Read the model definition and answer for the solid it produces. Units are mm, in the model's axes. A direction names the side the tool comes from. Coordinates: 2 decimals unless noted, no trailing zeros. Order: outer loops, then holes, each group sorted by start corner. A loop starts at its lowest first (then second) coordinate and runs counter-clockwise, first axis right, second up. Notation, with made-up numbers: (48, -11) -> (105, -11) arc R16 ccw to (105, 6) -> close; hole circle Ø8 at (-32.5, 54). An arc over 180 degrees is marked (long way). Use CSV: the item, a comma, the result in double quotes.
```python
from build123d import *

# Parameters (mm, degrees)
SKETCH_1_W      = 23
SKETCH_1_H      = 14
SKETCH_1_W_2    = 2
SKETCH_1_W_3    = 0.7
SKETCH_1_H_2    = 0.7
EXTRUDE_1_DEPTH = 1
SKETCH_1_3_W    = 2
SKETCH_1_3_H    = 14
SKETCH_1_3_W_2  = 0.7
SKETCH_1_3_H_2  = 0.7
EXTRUDE_2_DEPTH = 2
SKETCH_1_4_W    = 0.7
SKETCH_1_4_H    = 0.7
EXTRUDE_3_DEPTH = 2.5
SKETCH_1_5_W    = 0.7
SKETCH_1_5_H    = 0.7
EXTRUDE_4_DEPTH = 4
SKETCH_2_W      = 0.7
SKETCH_2_H      = 0.7
EXTRUDE_5_DEPTH = 7
SKETCH_4_W      = 19
SKETCH_4_H      = 12
EXTRUDE_6_DEPTH = 2.5
SKETCH_4_2_W    = 19
SKETCH_4_2_H    = 12
EXTRUDE_7_DEPTH = 1.5


with BuildPart() as part:
    # Sketch 1 → Extrude 1 (new body)
    # profile 1 of 7: a face of its own
    with BuildSketch(Plane.XY):
        with Locations((-13.5, 7)):
            Rectangle(SKETCH_1_W, SKETCH_1_H)
    # profile 2 of 7: a face of its own
    with BuildSketch(Plane.XY):
        with Locations((-1, 7)):
            Rectangle(SKETCH_1_W_2, SKETCH_1_H)
        with Locations((-1, 2)):
            Rectangle(SKETCH_1_W_3, SKETCH_1_H_2, mode=Mode.SUBTRACT)
        with Locations((-1, 4.5)):
            Rectangle(SKETCH_1_W_3, SKETCH_1_H_2, mode=Mode.SUBTRACT)
        with Locations((-1, 7)):
            Rectangle(SKETCH_1_W_3, SKETCH_1_H_2, mode=Mode.SUBTRACT)
        with Locations((-1, 9.5)):
            Rectangle(SKETCH_1_W_3, SKETCH_1_H_2, mode=Mode.SUBTRACT)
        with Locations((-1, 12)):
            Rectangle(SKETCH_1_W_3, SKETCH_1_H_2, mode=Mode.SUBTRACT)
    # profile 3 of 7: a face of its own
    with BuildSketch(Plane.XY):
        with Locations((-1, 12)):
            Rectangle(SKETCH_1_W_3, SKETCH_1_H_2)
    # profile 4 of 7: a face of its own
    with BuildSketch(Plane.XY):
        with Locations((-1, 9.5)):
            Rectangle(SKETCH_1_W_3, SKETCH_1_H_2)
    # profile 5 of 7: a face of its own
    with BuildSketch(Plane.XY):
        with Locations((-1, 7)):
            Rectangle(SKETCH_1_W_3, SKETCH_1_H_2)
    # profile 6 of 7: a face of its own
    with BuildSketch(Plane.XY):
        with Locations((-1, 4.5)):
            Rectangle(SKETCH_1_W_3, SKETCH_1_H_2)
    # profile 7 of 7: a face of its own
    with BuildSketch(Plane.XY):
        with Locations((-1, 2)):
            Rectangle(SKETCH_1_W_3, SKETCH_1_H_2)
    extrude(amount=EXTRUDE_1_DEPTH)

    # Sketch 1_3 → Extrude 2 (add)
    with BuildSketch(Plane.XY):
        with Locations((-1, 7)):
            Rectangle(SKETCH_1_3_W, SKETCH_1_3_H)
        with Locations((-1, 2)):
            Rectangle(SKETCH_1_3_W_2, SKETCH_1_3_H_2, mode=Mode.SUBTRACT)
        with Locations((-1, 4.5)):
            Rectangle(SKETCH_1_3_W_2, SKETCH_1_3_H_2, mode=Mode.SUBTRACT)
        with Locations((-1, 7)):
            Rectangle(SKETCH_1_3_W_2, SKETCH_1_3_H_2, mode=Mode.SUBTRACT)
        with Locations((-1, 9.5)):
            Rectangle(SKETCH_1_3_W_2, SKETCH_1_3_H_2, mode=Mode.SUBTRACT)
        with Locations((-1, 12)):
            Rectangle(SKETCH_1_3_W_2, SKETCH_1_3_H_2, mode=Mode.SUBTRACT)
    extrude(amount=-EXTRUDE_2_DEPTH)

    # Sketch 1_4 → Extrude 3 (add)
    with BuildSketch(Plane.XY):
        with Locations((-1, 12)):
            Rectangle(SKETCH_1_4_W, SKETCH_1_4_H)
        with Locations((-1, 9.5)):
            Rectangle(SKETCH_1_4_W, SKETCH_1_4_H)
        with Locations((-1, 7)):
            Rectangle(SKETCH_1_4_W, SKETCH_1_4_H)
        with Locations((-1, 4.5)):
            Rectangle(SKETCH_1_4_W, SKETCH_1_4_H)
        with Locations((-1, 2)):
            Rectangle(SKETCH_1_4_W, SKETCH_1_4_H)
    extrude(amount=EXTRUDE_3_DEPTH)

    # Sketch 1_5 → Extrude 4 (add)
    with BuildSketch(Plane.XY):
        with Locations((-1, 12)):
            Rectangle(SKETCH_1_5_W, SKETCH_1_5_H)
        with Locations((-1, 9.5)):
            Rectangle(SKETCH_1_5_W, SKETCH_1_5_H)
        with Locations((-1, 7)):
            Rectangle(SKETCH_1_5_W, SKETCH_1_5_H)
        with Locations((-1, 4.5)):
            Rectangle(SKETCH_1_5_W, SKETCH_1_5_H)
        with Locations((-1, 2)):
            Rectangle(SKETCH_1_5_W, SKETCH_1_5_H)
    extrude(amount=-EXTRUDE_4_DEPTH)

    # Sketch 2 → Extrude 5 (add)
    with BuildSketch(Plane(origin=(-0.65, 0, 0), x_dir=(0, 0, -1), z_dir=(1, 0, 0))):
        with Locations((3.65, 12)):
            Rectangle(SKETCH_2_W, SKETCH_2_H)
        with Locations((3.65, 9.5)):
            Rectangle(SKETCH_2_W, SKETCH_2_H)
        with Locations((3.65, 7)):
            Rectangle(SKETCH_2_W, SKETCH_2_H)
        with Locations((3.65, 4.5)):
            Rectangle(SKETCH_2_W, SKETCH_2_H)
        with Locations((3.65, 2)):
            Rectangle(SKETCH_2_W, SKETCH_2_H)
    extrude(amount=EXTRUDE_5_DEPTH)



with BuildPart() as body_2:
    # Sketch 4 → Extrude 6 (new body)
    with BuildSketch(Plane(origin=(-0.189903087, 0, -2.170602221), x_dir=(-0.9961946980917455, 0, 0.08715574274765837), z_dir=(-0.08715574274765839, 0, -0.9961946980917457))):
        with Locations((31.404867452, 7)):
            Rectangle(SKETCH_4_W, SKETCH_4_H)
    extrude(amount=EXTRUDE_6_DEPTH)


with BuildPart() as part_1:
    add(part.part)

    add(body_2.part)  # Extrude 7 merges body 2
    # Sketch 4_2 → Extrude 7 (add)
    with BuildSketch(Plane(origin=(-0.189903087, 0, -2.170602221), x_dir=(-0.9961946980917455, 0, 0.08715574274765837), z_dir=(-0.08715574274765839, 0, -0.9961946980917457))):
        with Locations((31.404867452, 7)):
            Rectangle(SKETCH_4_2_W, SKETCH_4_2_H)
    extrude(amount=-EXTRUDE_7_DEPTH)


solid = part_1.part
```
Item 1: The mould has two halves that part along X. Classify faces 4 (the flat face through (-25, 13.5, 0.5)), 5 (the flat face through (-22.11, 6.92, -1.4)), 6 (the flat face through (-9.9, 14, 0.2)): +X half, -X half, draft (parallel to the pull), parting line (faces both ways), or undercut.
Return value:
face 4,"-X half"
face 5,"undercut"
face 6,"draft"
Item 2: A tool of negligible diameter and unlimited length cuts with its end or side. For faces 1 (the flat face through (0, 7, 0)), 2 (the flat face through (-25, 0.5, 0.5)), 3 (the flat face through (-31.21, 7.08, 2.05)), from which of +Z, -Z, +X, -X, +Y, -Y can it reach the whole face along a straight path? Write none if from no direction.
Return value:
face 1,"+Z, +X, +Y, -Y"
face 2,"+Z, -Z, -X, -Y"
face 3,"+Z, +Y, -Y"
Item 3: Find section A-A, the plane y = 11. Give the vertices of the cut face in (x, z).
Return value:
outline,"(-41.16, -1.1) -> (-22.23, -2.75) -> (-21.99, 0) -> (-2, 0) -> (-2, -2) -> (0, -2) -> (0, 1) -> (-21.9, 1) -> (-21.88, 1.23) -> (-40.81, 2.89) -> close"
Item 4: Find section B-B, the plane z = 1.75. Give the vertices of the cut face in (x, y).
Return value:
outline,"(-40.91, 1) -> (-27.79, 1) -> (-27.79, 13) -> (-40.91, 13) -> close; (-1.35, 1.65) -> (-0.65, 1.65) -> (-0.65, 2.35) -> (-1.35, 2.35) -> close; (-1.35, 4.15) -> (-0.65, 4.15) -> (-0.65, 4.85) -> (-1.35, 4.85) -> close; (-1.35, 6.65) -> (-0.65, 6.65) -> (-0.65, 7.35) -> (-1.35, 7.35) -> close; (-1.35, 9.15) -> (-0.65, 9.15) -> (-0.65, 9.85) -> (-1.35, 9.85) -> close; (-1.35, 11.65) -> (-0.65, 11.65) -> (-0.65, 12.35) -> (-1.35, 12.35) -> close"
Item 5: Straight lines are drawn through the part: line 1 along Y through (x, z) = (-36.5, 1.5); line 2 along Z through (x, y) = (-0.5, 1.5); line 3 along Z through (x, y) = (-18, 4.5). For each, find the intervals that lie inside material, in ascending order.
Return value:
line 1,"y = 1 to 13"
line 2,"z = -2 to 1"
line 3,"z = 0 to 1"
Item 6: Find section D-D, the plane x = -29. Give the vertices of the cut face in (y, z).
Return value:
outline,"(1, -2.16) -> (13, -2.16) -> (13, 1.86) -> (1, 1.86) -> close"
Item 7: Find section C-C, the plane x = -8. Give the vertices of the cut face in (y, z), then the cut area to 3 significant figures.
Return value:
outline,"(0, 0) -> (14, 0) -> (14, 1) -> (0, 1) -> close"
area,"14.0 mm^2"
Item 8: Each of these flat-tipped pins is pushed along its axis until it touches: P1, Ø1.6, axis at x = 3, z = -3, coming from the +Y side; P2, Ø4, axis at x = -28.5, z = -2.5, coming from the -Y side; P3, Ø0.6, axis at x = 3, y = 2, coming from the +Z side. Where does it stop, or does it pass through?
Return value:
P1,"stops at y = 12.35"
P2,"stops at y = 1"
P3,"stops at z = -3.3"
